Could you check a few things on this model? Use its own coordinates, in mm. Coordinates: 2 decimals unless noted, no trailing zeros. Loops run counter-clockwise (first coordinate to the right, second up) from the corner with the lowest first, then second, coordinate; pieces in that order, holes last. Notation, with made-up numbers: M 20,81.5 L 47,81.5 A11 cw 47,89.5 Z; hole C 87,76.25 d5. An arc over 180 degrees is marked long. Use one line per item in the form item = value. Start each with the question number.
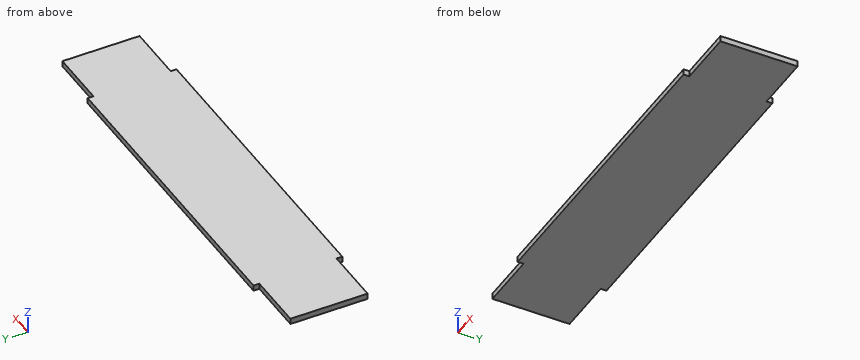
Solid Edge part; units mm, degrees
sketch "Sketch1" plane through (0, 0, 0) normal (0, 0, 1) x (1, 0, 0)
  line L0 (-110, -23) -> (110, -23)
  line L1 (110, -23) -> (110, 23)
  line L2 (110, 23) -> (-110, 23)
  line L3 (-110, 23) -> (-110, -23)
  dimension "D1" = 110
  dimension "D2" = 110
extrude "Ajout_matière_1" add sketch "Sketch1" along normal blind 3
sketch "Sketch2" plane through (0, 0, 3) normal (0, 0, 1) x (1, 0, 0)
  line L0 (-110, 23) -> (-80, 23)
  line L1 (-80, 23) -> (-80, 20)
  line L2 (-80, 20) -> (-110, 20)
  line L3 (-110, 20) -> (-110, 23)
  dimension "D1" = 110
  dimension "D2" = 110
extrude "Cutout1" cut sketch "Sketch2" against normal through all
mirror "Mirror1" about plane through (0, 0, 0) normal (1, 0, 0) of "Cutout1"
mirror "Mirror2" about plane through (0, 0, 0) normal (0, -1, 0) of "Mirror1", "Cutout1"
properties material "Acier S235"
Item 1: I want a section at A-A (z = 1.8). Write out the boundary of the cut face in (x, y).
Item 2: I'm going to push flat-ended pins straight in: P1, Ø1.5, axis at y = 21, z = 1, coming from the +X side; P2, Ø10, axis at x = 45.5, y = -9, coming from the -Z side; P3, Ø0.9, axis at x = 91.5, z = 2, coming from the +Y side; P4, Ø0.9, axis at x = -97.5, z = 1.5, coming from the -Y side. Where does each tip first touch, or does it pass through?
Item 3: Please list where this line runs through material, in increasing order: line 1 along Y through (x, z) = (-97, 2.7).
Item 4: I want a section at B-B (x = -95.5). Write out the boundary of the cut face in (y, z), plus the area to 3 significant figures.
Worked answers:
q1.outline = M -110,-20 L -80,-20 L -80,-23 L 80,-23 L 80,-20 L 110,-20 L 110,20 L 80,20 L 80,23 L -80,23 L -80,20 L -110,20 Z
q2.P1 = 80
q2.P2 = 0
q2.P3 = 20
q2.P4 = -20
q3.line_1 = -20 to 20
q4.outline = M -20,0 L 20,0 L 20,3 L -20,3 Z
q4.area = 120 mm²
